Design review of the part built by this model. Coordinates are the model's own, in mm. Face numbers are marked on the shaded views. A direction names the side the tool comes from. Give positions to 0.01 mm unless a question says otherwise; leave off trailing zeros. Write each loop counter-clockwise with the first axis right and the second up, starting at its lowest first coordinate (ties: lowest second). Pieces come first, ordered by that corner, then holes. Notation, with made-up numbers: (0.5, -10) -> (54.5, -10) arc R17 cw to (54.5, 16) -> close; hole circle Ø10 at (89.25, 82). An arc over 180 degrees is marked (long way). Use CSV: the item, a comma, the result in double quotes.
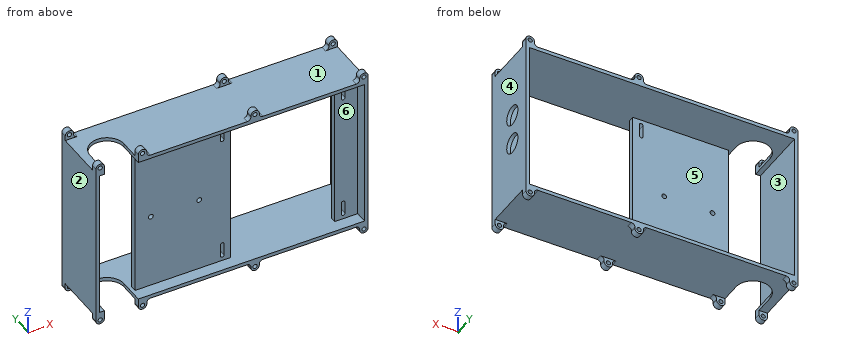
```python
from build123d import *

# Parameters (mm, degrees)
SKETCH1_W           = 225
SKETCH1_H           = 130
SKETCH1_W_2         = 219
SKETCH1_H_2         = 124
BOSS_EXTRUDE1_DEPTH = 50
CUT_EXTRUDE1_DEPTH  = 180.988888546
SKETCH4_R           = 1.75
BOSS_EXTRUDE2_DEPTH = 5
SKETCH6_R           = 8.15
CUT_EXTRUDE2_DEPTH  = 10
BOSS_EXTRUDE5_START = -5
SKETCH8_R           = 1.75
BOSS_EXTRUDE5_DEPTH = 5
BOSS_EXTRUDE6_START = -10
SKETCH9_W           = 19
SKETCH9_H           = 124
SKETCH9_W_2         = 14
BOSS_EXTRUDE6_DEPTH = 5
FILLET1_R           = 3
SKETCH10_W          = 124
SKETCH10_H          = 5
BOSS_EXTRUDE7_DEPTH = 65
SKETCH11_R          = 2
CUT_EXTRUDE3_DEPTH  = 140.560918598


with BuildPart() as part:
    # Sketch1 → Boss-Extrude1 (new body)
    with BuildSketch(Plane(origin=(0, 0, 0), x_dir=(1, 0, 0), z_dir=(0, 1, 0))):
        with Locations((1.5, 0)):
            Rectangle(SKETCH1_W, SKETCH1_H)
        with Locations((1.5, 0)):
            Rectangle(SKETCH1_W_2, SKETCH1_H_2, mode=Mode.SUBTRACT)
    extrude(amount=BOSS_EXTRUDE1_DEPTH)

    # Sketch3 → Cut-Extrude1 (cut, through all)
    with BuildSketch(Plane.XY.offset(65)):
        with BuildLine():
            Line((-104, 0), (-76, 0))
            Line((-76, 0), (-76, 21))
            ThreePointArc((-76, 21), (-90, 35), (-104, 21))
            Line((-104, 21), (-104, 0))
        make_face()
    extrude(amount=-CUT_EXTRUDE1_DEPTH, mode=Mode.SUBTRACT)

    # Sketch4 → Boss-Extrude2 (add)
    # profile 1 of 8: a face of its own
    with BuildSketch(Plane.XZ):
        with BuildLine():
            Line((-111, 69), (-111, 65))
            Line((-111, 65), (-104, 65))
            Line((-104, 65), (-104, 69))
            ThreePointArc((-104, 69), (-107.5, 72.5), (-111, 69))
        make_face()
        with Locations(Location((-107.5, 69, 0), (0, 0, 270))):
            Circle(SKETCH4_R, mode=Mode.SUBTRACT)
    # profile 2 of 8: a face of its own
    with BuildSketch(Plane.XZ):
        with BuildLine():
            Line((-76, 69), (-76, 65))
            Line((-76, 65), (-69, 65))
            Line((-69, 65), (-69, 69))
            ThreePointArc((-69, 69), (-72.5, 72.5), (-76, 69))
        make_face()
        with Locations(Location((-72.5, 69, 0), (0, 0, 270))):
            Circle(SKETCH4_R, mode=Mode.SUBTRACT)
    # profile 3 of 8: a face of its own
    with BuildSketch(Plane.XZ):
        with BuildLine():
            Line((-76, -65), (-69, -65))
            Line((-69, -65), (-69, -69))
            ThreePointArc((-69, -69), (-72.5, -72.5), (-76, -69))
            Line((-76, -69), (-76, -65))
        make_face()
        with Locations(Location((-72.5, -69, 0), (0, 0, 90))):
            Circle(SKETCH4_R, mode=Mode.SUBTRACT)
    # profile 4 of 8: a face of its own
    with BuildSketch(Plane.XZ):
        with BuildLine():
            Line((-111, -65), (-104, -65))
            Line((-104, -65), (-104, -69))
            ThreePointArc((-104, -69), (-107.5, -72.5), (-111, -69))
            Line((-111, -69), (-111, -65))
        make_face()
        with Locations(Location((-107.5, -69, 0), (0, 0, 90))):
            Circle(SKETCH4_R, mode=Mode.SUBTRACT)
    # profile 5 of 8: a face of its own
    with BuildSketch(Plane.XZ):
        with BuildLine():
            Line((17, -65), (24, -65))
            Line((24, -65), (24, -69))
            ThreePointArc((24, -69), (20.5, -72.5), (17, -69))
            Line((17, -69), (17, -65))
        make_face()
        with Locations(Location((20.5, -69, 0), (0, 0, 90))):
            Circle(SKETCH4_R, mode=Mode.SUBTRACT)
    # profile 6 of 8: a face of its own
    with BuildSketch(Plane.XZ):
        with BuildLine():
            Line((107, -65), (114, -65))
            Line((114, -65), (114, -69))
            ThreePointArc((114, -69), (110.5, -72.5), (107, -69))
            Line((107, -69), (107, -65))
        make_face()
        with Locations(Location((110.5, -69, 0), (0, 0, 90))):
            Circle(SKETCH4_R, mode=Mode.SUBTRACT)
    # profile 7 of 8: a face of its own
    with BuildSketch(Plane.XZ):
        with BuildLine():
            Line((17, 69), (17, 65))
            Line((17, 65), (24, 65))
            Line((24, 65), (24, 69))
            ThreePointArc((24, 69), (20.5, 72.5), (17, 69))
        make_face()
        with Locations(Location((20.5, 69, 0), (0, 0, 270))):
            Circle(SKETCH4_R, mode=Mode.SUBTRACT)
    # profile 8 of 8: a face of its own
    with BuildSketch(Plane.XZ):
        with BuildLine():
            Line((107, 69), (107, 65))
            Line((107, 65), (114, 65))
            Line((114, 65), (114, 69))
            ThreePointArc((114, 69), (110.5, 72.5), (107, 69))
        make_face()
        with Locations(Location((110.5, 69, 0), (0, 0, 270))):
            Circle(SKETCH4_R, mode=Mode.SUBTRACT)
    extrude(amount=-BOSS_EXTRUDE2_DEPTH)

    # Sketch6 → Cut-Extrude2 (cut)
    with BuildSketch(Plane(origin=(114, 0, 0), x_dir=(0, 0, -1), z_dir=(1, 0, 0))):
        with Locations((-12.75, 30)):
            Circle(SKETCH6_R)
        with Locations((12.75, 30)):
            Circle(SKETCH6_R)
    extrude(amount=-CUT_EXTRUDE2_DEPTH, mode=Mode.SUBTRACT)

    # Sketch8 → Boss-Extrude5 (add)
    # profile 1 of 6: a face of its own
    with BuildSketch(Plane(origin=(0, 50, 0), x_dir=(1, 0, 0), z_dir=(0, 1, 0)).offset(BOSS_EXTRUDE5_START)):
        with BuildLine():
            Line((114, 65), (107, 65))
            Line((107, 65), (107, 69))
            ThreePointArc((107, 69), (110.5, 72.5), (114, 69))
            Line((114, 69), (114, 65))
        make_face()
        with Locations(Location((110.5, 69, 0), (0, 0, 270))):
            Circle(SKETCH8_R, mode=Mode.SUBTRACT)
    # profile 2 of 6: a face of its own
    with BuildSketch(Plane(origin=(0, 50, 0), x_dir=(1, 0, 0), z_dir=(0, 1, 0)).offset(BOSS_EXTRUDE5_START)):
        with BuildLine():
            Line((114, -65), (114, -69))
            ThreePointArc((114, -69), (110.5, -72.5), (107, -69))
            Line((107, -69), (107, -65))
            Line((107, -65), (114, -65))
        make_face()
        with Locations(Location((110.5, -69, 0), (0, 0, 90))):
            Circle(SKETCH8_R, mode=Mode.SUBTRACT)
    # profile 3 of 6: a face of its own
    with BuildSketch(Plane(origin=(0, 50, 0), x_dir=(1, 0, 0), z_dir=(0, 1, 0)).offset(BOSS_EXTRUDE5_START)):
        with BuildLine():
            Line((-104, 65), (-111, 65))
            Line((-111, 65), (-111, 69))
            ThreePointArc((-111, 69), (-107.5, 72.5), (-104, 69))
            Line((-104, 69), (-104, 65))
        make_face()
        with Locations(Location((-107.5, 69, 0), (0, 0, 270))):
            Circle(SKETCH8_R, mode=Mode.SUBTRACT)
    # profile 4 of 6: a face of its own
    with BuildSketch(Plane(origin=(0, 50, 0), x_dir=(1, 0, 0), z_dir=(0, 1, 0)).offset(BOSS_EXTRUDE5_START)):
        with BuildLine():
            Line((24, 65), (17, 65))
            Line((17, 65), (17, 69))
            ThreePointArc((17, 69), (20.5, 72.5), (24, 69))
            Line((24, 69), (24, 65))
        make_face()
        with Locations(Location((20.5, 69, 0), (0, 0, 270))):
            Circle(SKETCH8_R, mode=Mode.SUBTRACT)
    # profile 5 of 6: a face of its own
    with BuildSketch(Plane(origin=(0, 50, 0), x_dir=(1, 0, 0), z_dir=(0, 1, 0)).offset(BOSS_EXTRUDE5_START)):
        with BuildLine():
            Line((24, -65), (24, -69))
            ThreePointArc((24, -69), (20.5, -72.5), (17, -69))
            Line((17, -69), (17, -65))
            Line((17, -65), (24, -65))
        make_face()
        with Locations(Location((20.5, -69, 0), (0, 0, 90))):
            Circle(SKETCH8_R, mode=Mode.SUBTRACT)
    # profile 6 of 6: a face of its own
    with BuildSketch(Plane(origin=(0, 50, 0), x_dir=(1, 0, 0), z_dir=(0, 1, 0)).offset(BOSS_EXTRUDE5_START)):
        with BuildLine():
            Line((-111, -65), (-104, -65))
            Line((-104, -65), (-104, -69))
            ThreePointArc((-104, -69), (-107.5, -72.5), (-111, -69))
            Line((-111, -69), (-111, -65))
        make_face()
        with Locations(Location((-107.5, -69, 0), (0, 0, 90))):
            Circle(SKETCH8_R, mode=Mode.SUBTRACT)
    extrude(amount=BOSS_EXTRUDE5_DEPTH)

    # Sketch9 → Boss-Extrude6 (add)
    # profile 1 of 2: a face of its own
    with BuildSketch(Plane.XZ.offset(BOSS_EXTRUDE6_START)):
        with Locations((101.5, 0)):
            Rectangle(SKETCH9_W, SKETCH9_H)
        with BuildLine():
            Line((97.5, 57.5), (97.5, 47.5))
            ThreePointArc((97.5, 47.5), (99, 46), (100.5, 47.5))
            Line((100.5, 47.5), (100.5, 57.5))
            ThreePointArc((100.5, 57.5), (99, 59), (97.5, 57.5))
        make_face(mode=Mode.SUBTRACT)
        with BuildLine():
            Line((100.5, -47.5), (100.5, -57.5))
            ThreePointArc((100.5, -57.5), (99, -59), (97.5, -57.5))
            Line((97.5, -57.5), (97.5, -47.5))
            ThreePointArc((97.5, -47.5), (99, -46), (100.5, -47.5))
        make_face(mode=Mode.SUBTRACT)
    # profile 2 of 2: a face of its own
    with BuildSketch(Plane.XZ.offset(BOSS_EXTRUDE6_START)):
        with Locations((-1, 0)):
            Rectangle(SKETCH9_W_2, SKETCH9_H)
        with BuildLine():
            Line((-2.5, 57.5), (-2.5, 47.5))
            ThreePointArc((-2.5, 47.5), (-1, 46), (0.5, 47.5))
            Line((0.5, 47.5), (0.5, 57.5))
            ThreePointArc((0.5, 57.5), (-1, 59), (-2.5, 57.5))
        make_face(mode=Mode.SUBTRACT)
        with BuildLine():
            Line((-2.5, -47.5), (-2.5, -57.5))
            ThreePointArc((-2.5, -57.5), (-1, -59), (0.5, -57.5))
            Line((0.5, -57.5), (0.5, -47.5))
            ThreePointArc((0.5, -47.5), (-1, -46), (-2.5, -47.5))
        make_face(mode=Mode.SUBTRACT)
    extrude(amount=-BOSS_EXTRUDE6_DEPTH)

    # Fillet1
    fillet1_edges = [part.edges().sort_by_distance(p)[0] for p in [
        (17, 2.5, -65),
        (24, 2.5, -65),
        (107, 2.5, -65),
        (24, 2.5, 65),
        (17, 2.5, 65),
        (107, 2.5, 65),
        (107, 47.5, -65),
        (107, 47.5, 65),
        (-104, 47.5, -65),
        (24, 47.5, -65),
        (17, 47.5, -65),
        (17, 47.5, 65),
        (24, 47.5, 65),
        (-104, 47.5, 65),
        (-69, 2.5, 65),
        (-69, 2.5, -65),
    ]]
    fillet(fillet1_edges, radius=FILLET1_R)

    # Sketch10 → Boss-Extrude7 (add)
    with BuildSketch(Plane.ZY.offset(8)):
        with Locations((0, 12.5)):
            Rectangle(SKETCH10_W, SKETCH10_H)
    extrude(amount=BOSS_EXTRUDE7_DEPTH)

    # Sketch11 → Cut-Extrude3 (cut, through all)
    with BuildSketch(Plane(origin=(0, 15, 0), x_dir=(1, 0, 0), z_dir=(0, 1, 0))):
        with Locations(Location((-60, 0, 0), (0, 0, 270))):
            Circle(SKETCH11_R)
        with Locations(Location((-20, 0, 0), (0, 0, 270))):
            Circle(SKETCH11_R)
    extrude(amount=-CUT_EXTRUDE3_DEPTH, mode=Mode.SUBTRACT)


solid = part.part
```
(1) Take a section at D-D (z = 10.5). Write out the cut boundary in (x, y).
Established:
outline,"(-111, 0) -> (-108, 0) -> (-108, 50) -> (-111, 50) -> close; (-73, 10) -> (6, 10) -> (6, 15) -> (-73, 15) -> close; (92, 10) -> (111, 10) -> (111, 0) -> (114, 0) -> (114, 22.17) -> (111, 22.17) -> (111, 15) -> (92, 15) -> close; (111, 37.83) -> (114, 37.83) -> (114, 50) -> (111, 50) -> close"
(2) Mouldability with a two-part tool opening along Z and no side actions: class the marked faces 1, 2 and 3 as +Z half, -Z half, draft (parallel to the pull), parting line (faces both ways), or undercut.
Established:
face 1,"+Z half"
face 2,"draft"
face 3,"undercut"
(3) Take a section at A-A (z = -12.75). Write out the cut boundary in (x, y), then the cut area to 3 significant figures.
Established:
outline,"(-111, 0) -> (-108, 0) -> (-108, 50) -> (-111, 50) -> close; (-73, 10) -> (6, 10) -> (6, 15) -> (-73, 15) -> close; (92, 10) -> (111, 10) -> (111, 0) -> (114, 0) -> (114, 21.85) -> (111, 21.85) -> (111, 15) -> (92, 15) -> close; (111, 38.15) -> (114, 38.15) -> (114, 50) -> (111, 50) -> close"
area,"741 mm2"
(4) Take a section at C-C (x = -11.5). Write out the cut boundary in (y, z).
Established:
outline,"(0, -65) -> (50, -65) -> (50, -62) -> (15, -62) -> (15, 62) -> (50, 62) -> (50, 65) -> (0, 65) -> (0, 62) -> (10, 62) -> (10, -62) -> (0, -62) -> close"
(5) Clearance check with flat-ended pins moving along their axes: pin 1 (1 mm diameter, centred on x = 80.5, y = 11.5, fed in from -Z); pin 2 (1.5 mm diameter, centred on x = -7.5, z = 35.5, fed in from +Y). State where each tip first meets the part, or that it passes through.
Established:
pin 1,"stops at z = -65"
pin 2,"stops at y = 15"
(6) For line 1 along X through (y, z) = (48.3, 69); line 2 along Z through (x, y) = (-107.5, 47.6); line 3 along X through (y, z) = (6, -34), list the stretches that pass through material, from the lowest coordinate up. Write a range as [from, to].
Established:
line 1,"x = [-111, -109.25], [-105.75, -104], [17, 18.75], [22.25, 24], [107, 108.75], [112.25, 114]"
line 2,"z = [-72.5, -70.75], [-67.25, -62], [62, 67.25], [70.75, 72.5]"
line 3,"x = [-111, -108], [111, 114]"
(7) Tool access review of the marked faces 4, 5 and 6: name each direction out of +Z, -Z, +X, -X, +Y, -Y from which nothing blocks a thin tool from reaching the whole face with its end or side.
Established:
face 4,"+Z, -Z, +X, +Y, -Y"
face 5,"+Y"
face 6,"-Y"
(8) Take a section at B-B (x = 75). Write out the cut boundary in (y, z).
Established:
outline,"(0, -65) -> (50, -65) -> (50, -62) -> (0, -62) -> close; (0, 62) -> (50, 62) -> (50, 65) -> (0, 65) -> close"
